The listing builds one solid part. Answer for the finished solid, in the listing's coordinates (mm). A direction names the side the tool comes from. Coordinates: 2 decimals unless noted, no trailing zeros. Order: outer loops, then holes, each group sorted by start corner. A loop starts at its lowest first (then second) coordinate and runs counter-clockwise, first axis right, second up. Notation, with made-up numbers: (-32.5, -12.5) -> (9.5, -12.5) arc R25 cw to (9.5, 25.5) -> close; hole circle Ø9 at (-33, 49.5). An arc over 180 degrees is marked (long way). Answer in a Markdown table with one row per item.
```python
from build123d import *

# Parameters (mm, degrees)
SKETCH1_R           = 14
BOSS_EXTRUDE1_DEPTH = 1
SKETCH2_R           = 11.5
BOSS_EXTRUDE2_DEPTH = 7
SKETCH3_R           = 14
BOSS_EXTRUDE3_DEPTH = 1
SKETCH4_R           = 9
BOSS_EXTRUDE4_DEPTH = 6
SKETCH5_R           = 4
CUT_EXTRUDE1_DEPTH  = 23
CHAMFER1_SIZE       = 0.5


with BuildPart() as part:
    # Sketch1 → Boss-Extrude1 (new body)
    with BuildSketch(Plane.XY):
        Circle(SKETCH1_R)
    extrude(amount=BOSS_EXTRUDE1_DEPTH)

    # Sketch2 → Boss-Extrude2 (add)
    with BuildSketch(Plane.XY.offset(1)):
        Circle(SKETCH2_R)
    extrude(amount=BOSS_EXTRUDE2_DEPTH)

    # Sketch3 → Boss-Extrude3 (add)
    with BuildSketch(Plane.XY.offset(8)):
        Circle(SKETCH3_R)
    extrude(amount=BOSS_EXTRUDE3_DEPTH)

    # Sketch4 → Boss-Extrude4 (add)
    with BuildSketch(Plane.XY.offset(9)):
        Circle(SKETCH4_R)
    extrude(amount=BOSS_EXTRUDE4_DEPTH)

    # Sketch5 → Cut-Extrude1 (cut)
    with BuildSketch(Plane(origin=(0, 0, 0), x_dir=(-1, 0, 0), z_dir=(0, 0, -1))):
        Circle(SKETCH5_R)
    extrude(amount=-CUT_EXTRUDE1_DEPTH, mode=Mode.SUBTRACT)

    # Chamfer1
    chamfer1_edges = [part.edges().sort_by_distance(p)[0] for p in [
        (-9, 0, 15),
        (4, 0, 15),
        (4, 0, 0),
    ]]
    chamfer(chamfer1_edges, length=CHAMFER1_SIZE)


solid = part.part
```
(1) For a pull along X with two mould halves and no side action, classify faces 4 (the cylindrical face through (12.932, -5.362, 0.493)), 5 (the flat face through (2, 11.5, 8)), 6 (the cylindrical face through (0.867, -3.905, 7.402)) as released by +X, released by -X, zero draft, split by the parting line, or undercut.
Check values:
| item | result |
|---|---|
| face 4 | split by the parting line |
| face 5 | zero draft |
| face 6 | undercut |
(2) A cutting plane is placed at A-A, the plane x = 0. Determine the outline of the cut face in (y, z), then the cut area to 3 significant figures.
Check values:
| item | result |
|---|---|
| outline | (-14, 0) -> (-4.5, 0) -> (-4, 0.5) -> (-4, 14.5) -> (-4.5, 15) -> (-8.5, 15) -> (-9, 14.5) -> (-9, 9) -> (-14, 9) -> (-14, 8) -> (-11.5, 8) -> (-11.5, 1) -> (-14, 1) -> close; (4, 0.5) -> (4.5, 0) -> (14, 0) -> (14, 1) -> (11.5, 1) -> (11.5, 8) -> (14, 8) -> (14, 9) -> (9, 9) -> (9, 14.5) -> (8.5, 15) -> (4.5, 15) -> (4, 14.5) -> close |
| area | 204 mm² |
(3) Which of the six approach directions +Z, -Z, +X, -X, +Y, -Y give full straight-line access (tool end or side, diameter ignored) to faces 1 (the flat face through (3, -9, 9)), 2 (the flat face through (4, -4, 15)), 3 (the cylindrical face through (-1.5, 11.4, 4.5))?
Check values:
| item | result |
|---|---|
| face 1 | +Z |
| face 2 | +Z, +X, -X, +Y, -Y |
| face 3 | none |
(4) Find the intervals of material crossed by line 1 along X through (y, z) = (0.25, 2.5); line 2 along Y through (x, z) = (0, 11); line 3 along Z through (x, y) = (-4.5, 11.75), in increasing order. Write a range as from..to.
Check values:
| item | result |
|---|---|
| line 1 | -11.5..-3.99, 3.99..11.5 |
| line 2 | -9..-4, 4..9 |
| line 3 | 0..1, 8..9 |
(5) Flat-ended cylindrical pins translate along their axes: pin 1 (2 mm diameter, centred on y = -0.5, z = 4, fed in from +X); pin 2 (3 mm diameter, centred on x = 0.5, z = 4.5, fed in from -Y). Find the tip coordinate at first contact, or state that the pin passes through.
Check values:
| item | result |
|---|---|
| pin 1 | x = 11.5 |
| pin 2 | y = -11.5 |
(6) A cutting plane is placed at C-C, the plane z = 12.75. Determine the outline of the cut face in (x, y), then the cut area to 3 significant figures.
Check values:
| item | result |
|---|---|
| outline | circle Ø18 at (0, 0); hole circle Ø8 at (0, 0) |
| area | 204 mm² |
(7) A cutting plane is placed at D-D, the plane x = -10.5. Determine the outline of the cut face in (y, z), then the cut area to 3 significant figures.
Check values:
| item | result |
|---|---|
| outline | (-9.26, 0) -> (9.26, 0) -> (9.26, 1) -> (4.69, 1) -> (4.69, 8) -> (9.26, 8) -> (9.26, 9) -> (-9.26, 9) -> (-9.26, 8) -> (-4.69, 8) -> (-4.69, 1) -> (-9.26, 1) -> close |
| area | 103 mm² |
